Could you check a few things on this model? Use its own coordinates, in mm. Face numbers are marked on the shaded views. A direction names the side the tool comes from. Give positions to 0.01 mm unless a question says otherwise; leave off trailing zeros. Order: outer loops, then holes, each group sorted by start corner. A loop starts at its lowest first (then second) coordinate and runs counter-clockwise, first axis right, second up.
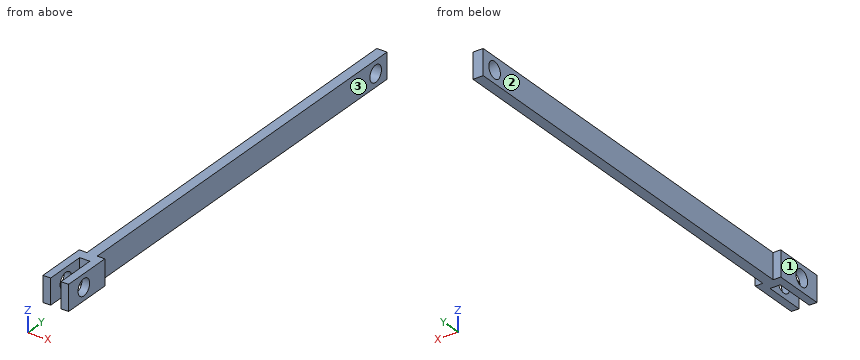
from build123d import *

# Parameters (mm, degrees)
F0_W          = 400
F0_H          = 25
F1_DEPTH      = 5
F1_DEPTH_BACK = 5
F2_W          = 7.5
F2_H          = 25
F2_W_2        = 10
F3_DEPTH      = 10
F4_W          = 7.5
F4_H          = 25
F5_DEPTH      = 40
F6_R          = 8
F7_DEPTH      = 25
F8_R          = 8
F9_DEPTH      = 25
F10_R         = 8
F11_DEPTH     = 25


with BuildPart() as f1:
    # F0 (on Right) → F1 (new body, two sides)
    with BuildSketch(Plane.YZ) as f1_sk:
        Rectangle(F0_W, F0_H)
    extrude(amount=F1_DEPTH)
    extrude(f1_sk.sketch, amount=-F1_DEPTH_BACK)

    # F2 (on face) → F3 (join)
    with BuildSketch(Plane.XZ.offset(200)):
        with Locations((-8.75, 0)):
            Rectangle(F2_W, F2_H)
        Rectangle(F2_W_2, F2_H)
        with Locations((8.75, 0)):
            Rectangle(F2_W, F2_H)
    extrude(amount=F3_DEPTH)

    # F4 (on face) → F5 (join)
    with BuildSketch(Plane.XZ.offset(210)):
        with Locations((8.75, 0)):
            Rectangle(F4_W, F4_H)
        with Locations((-8.75, 0)):
            Rectangle(F4_W, F4_H)
    extrude(amount=F5_DEPTH)

    # F6 (on face) → F7 (cut)
    with BuildSketch(Plane.YZ.offset(12.5)):
        with Locations((-228.9973199368, 0)):
            Circle(F6_R)
    extrude(amount=-F7_DEPTH, mode=Mode.SUBTRACT)

    # F8 (on face) → F9 (cut)
    with BuildSketch(Plane.YZ.offset(5)):
        with Locations((234.8896563053, 0)):
            Circle(F8_R)
    extrude(amount=-F9_DEPTH, mode=Mode.SUBTRACT)

    # F10 (on face) → F11 (cut)
    with BuildSketch(Plane.YZ.offset(5)):
        with Locations((184.34253335, 0)):
            Circle(F10_R)
    extrude(amount=-F11_DEPTH, mode=Mode.SUBTRACT)


solid = f1.part
Item 1: For pin 1 (9.5 mm diameter, centred on y = 184.34, z = 0, fed in from -X); pin 2 (10 mm diameter, centred on y = 154, z = -1.5, fed in from -X); pin 3 (6 mm diameter, centred on x = 10, z = 0.5, fed in from +Y); pin 4 (10 mm diameter, centred on y = -157, z = -0.5, fed in from +X), each with a flat end and sliding along its axis, tell me the tip position at first contact or that it passes through.
Findings:
pin 1: passes through
pin 2: stops at x = -5
pin 3: stops at y = -200
pin 4: stops at x = 5
Item 2: Imagine slicing it at C-C on y = -31.5. List the corners of the cut face in (x, z) for me.
Findings:
outline: (-5, -12.5) - (5, -12.5) - (5, 12.5) - (-5, 12.5) - close
Item 3: For the marked faces 1, 2 and 3, which set-ups out of +Z, -Z, +X, -X, +Y, -Y let a thin tool reach every point of the face, with its end or its side?
Findings:
face 1: +Z, -Z, -X, +Y, -Y
face 2: +Z, -Z, -X, +Y
face 3: +Z, -Z, +X, +Y
Item 4: Imagine slicing it at A-A on z = 0. List the corners of the cut face in (x, y) for me.
Findings:
outline: (-12.5, -250) - (-5, -250) - (-5, -237) - (-12.5, -237) - close; (-12.5, -221) - (-5, -221) - (-5, -210) - (5, -210) - (5, -221) - (12.5, -221) - (12.5, -200) - (5, -200) - (5, 176.34) - (-5, 176.34) - (-5, -200) - (-12.5, -200) - close; (-5, 192.34) - (5, 192.34) - (5, 200) - (-5, 200) - close; (5, -250) - (12.5, -250) - (12.5, -237) - (5, -237) - close
Item 5: Please list where these lines run through material, in increasing order: line 1 along X through (y, z) = (-154, 0.5); line 2 along Y through (x, z) = (-11.5, 8.25); line 3 along Y through (x, z) = (5.25, -6.25).
Findings:
line 1: x = -5 to 5
line 2: y = -250 to -200
line 3: y = -250 to -233.99, -224 to -200
Item 6: Imagine slicing it at B-B on x = 0.25. List the corners of the cut face in (y, z) for me, then the cut area to 3 significant figures.
Findings:
outline: (-210, -12.5) - (200, -12.5) - (200, 12.5) - (-210, 12.5) - close; hole circle Ø16 at (184.34, 0)
area: 10,000 mm2
